```python
from build123d import *

# Parameters (mm, degrees)
SKETCH_1_R          = 2.05
SKETCH_1_R_2        = 9.525
SKETCH_1_W          = 2.1
SKETCH_1_H          = 8.1
EXTRUDE_1_DEPTH     = 2
FILLET_1_R          = 2
SKETCH_3_R          = 2.05
SKETCH_3_R_2        = 2
SKETCH_3_W          = 8.2
SKETCH_3_H          = 2.2
CUT_EXTRUDE_1_DEPTH = 2
FILLET_2_R          = 2


with BuildPart() as part:
    # 草图1 → 凸台-拉伸1 (new body)
    with BuildSketch(Plane.XY):
        with BuildLine():
            Line((230.542857143, -30.045714286), (199.556073527, -36.55591431))
            Line((199.556073527, -36.55591431), (192.746868021, -38.145714286))
            Line((192.746868021, -38.145714286), (21.365844759, -38.145714286))
            Line((21.365844759, -38.145714286), (2.692857143, -38.295714286))
            Line((2.692857143, -38.295714286), (2.692857143, -35.802553436))
            Line((2.692857143, -35.802553436), (-5.457142857, -35.802553436))
            Line((-5.457142857, -35.802553436), (-5.457142857, 41.704285714))
            Line((-5.457142857, 41.704285714), (7.542857143, 41.704285714))
            Line((7.542857143, 41.704285714), (7.542857143, 14.854285714))
            Line((7.542857143, 14.854285714), (16.542857143, 14.854285714))
            Line((16.542857143, 14.854285714), (16.542857143, 41.704285714))
            Line((16.542857143, 41.704285714), (199.542857143, 41.704285714))
            Line((199.542857143, 41.704285714), (230.542857143, 29.754285714))
            ThreePointArc((230.542857143, 29.754285714), (260.442857143, -0.145714286), (230.542857143, -30.045714286))
        make_face()
        with Locations((0.542857143, 29.854285714)):
            Circle(SKETCH_1_R, mode=Mode.SUBTRACT)
        with Locations((0.542857143, -0.145714286)):
            Circle(SKETCH_1_R, mode=Mode.SUBTRACT)
        with Locations((0.542857143, -30.145714286)):
            Circle(SKETCH_1_R, mode=Mode.SUBTRACT)
        with Locations((230.542857143, -0.145714286)):
            Circle(SKETCH_1_R_2, mode=Mode.SUBTRACT)
        with Locations((0.542857143, 14.854285714)):
            Rectangle(SKETCH_1_W, SKETCH_1_H, mode=Mode.SUBTRACT)
        with BuildLine():
            Line((59.099206329, 22.4106349), (50.542857143, 30.966984086))
            Line((50.542857143, 30.966984086), (19.430158771, -0.145714286))
            Line((19.430158771, -0.145714286), (50.542857143, -31.258412658))
            Line((50.542857143, -31.258412658), (81.655555515, -0.145714286))
            Line((81.655555515, -0.145714286), (73.099206329, 8.4106349))
            ThreePointArc((73.099206329, 8.4106349), (74.584487703, 23.895916275), (59.099206329, 22.4106349))
        make_face(mode=Mode.SUBTRACT)
        with Locations((0.542857143, -15.145714286)):
            Rectangle(SKETCH_1_W, SKETCH_1_H, mode=Mode.SUBTRACT)
    extrude(amount=EXTRUDE_1_DEPTH)

    # 圆角1
    fillet_1_edges = [part.edges().sort_by_distance(p)[0] for p in [
        (7.542857143, 41.704285714, 1),
        (7.542857143, 14.854285714, 1),
        (16.542857143, 14.854285714, 1),
        (16.542857143, 41.704285714, 1),
    ]]
    fillet(fillet_1_edges, radius=FILLET_1_R)

    # 草图3 → 切除-拉伸1 (cut)
    with BuildSketch(Plane.XY.offset(2)):
        with Locations((25.542857143, 35.704285714)):
            Circle(SKETCH_3_R)
        with Locations((110.542857143, 35.704285714)):
            Circle(SKETCH_3_R)
        with Locations((195.542857143, 35.704285714)):
            Circle(SKETCH_3_R)
        with Locations((110.542857143, -34.295714286)):
            Circle(SKETCH_3_R)
        with Locations((195.542857143, -34.295714286)):
            Circle(SKETCH_3_R)
        with Locations((25.542857143, -34.295714286)):
            Circle(SKETCH_3_R)
        with Locations((190.542857143, -0.145714286)):
            Circle(SKETCH_3_R_2)
        with Locations((140.542857143, 16.354285714)):
            Circle(SKETCH_3_R_2)
        with Locations(Location((140.542857143, -16.645714286, 0), (0, 0, 180))):
            Circle(SKETCH_3_R_2)
        with Locations((199.574018739, 19.704285714)):
            Circle(SKETCH_3_R)
        Polygon((148.153334198, 25.704285714), (148.153334198, 9.632158315), (167.669488896, 25.704285714), align=None)
        Polygon((185.542857143, -24.295714286), (138.41622539, -24.295714286), (185.542857143, 14.51445304), align=None)
        Polygon((120.542857143, -13.105881612), (120.542857143, 25.704285714), (134.014872528, 25.704285714), (134.014872528, -2.011280706), align=None)
        with Locations((184.574018739, 19.704285714)):
            Rectangle(SKETCH_3_W, SKETCH_3_H)
    extrude(amount=-CUT_EXTRUDE_1_DEPTH, mode=Mode.SUBTRACT)

    # 圆角2
    fillet_2_edges = [part.edges().sort_by_distance(p)[0] for p in [
        (167.669488896, 25.704285714, 1),
        (148.153334198, 9.632158315, 1),
        (148.153334198, 25.704285714, 1),
        (120.542857143, 25.704285714, 1),
        (134.014872528, 25.704285714, 1),
        (134.014872528, -2.011280706, 1),
        (120.542857143, -13.105881612, 1),
        (185.542857143, 14.51445304, 1),
        (185.542857143, -24.295714286, 1),
        (138.41622539, -24.295714286, 1),
    ]]
    fillet(fillet_2_edges, radius=FILLET_2_R)


solid = part.part
```
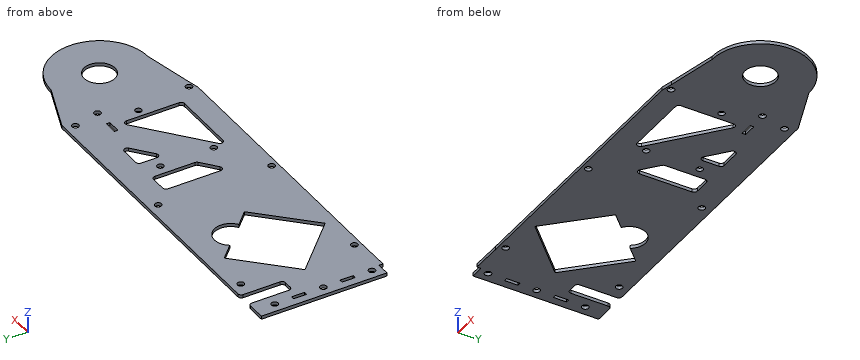
Can you work these out from the model? Positions are in its coordinate system, mm. Coordinates: 2 decimals unless noted, no trailing zeros. Write each loop counter-clockwise with the first axis right and the second up, starting at its lowest first coordinate (ties: lowest second). Pieces come first, ordered by that corner, then holes. Notation, with made-up numbers: M 5,62.25 L 10,62.25 A27 cw 10,93.25 Z; hole C -28,-32.5 d5. An arc over 180 degrees is marked long. Write item = value, one per line. Start each with the question number.
Q1. If we section it at C-C, the plane x = 218.5: Write out the boundary of the cut face in (y, z).
Q2. If we section it at B-B, the plane z = 1.6: State how many separate pieces and enclosed holes the cut face has, then the cut area to 3 significant figures.
Q3. If we section it at A-A, the plane x = 46: Write out the boundary of the cut face in (y, z), then the cut area to 3 significant figures.
Q4. I'm going to push flat-ended pins straight in: pin 1 (12 mm diameter, centred on x = 47.5, y = 27.5, fed in from -Z); pin 2 (3.5 mm diameter, centred on x = 110.54, y = 35.7, fed in from +Z); pin 3 (1 mm diameter, centred on x = 0.5, z = 1, fed in from -Y); pin 4 (0.6 mm diameter, centred on y = -37.5, z = 1.5, fed in from -X). Where does each tip first touch, or does it pass through?
Q5. If I drill on L1, parallel to X at y = 22, z = 1.7; L2, parallel to X at y = 2.5, z = 1.3; L3, parallel to X at y = -22.5, z = 0.4, over which ranges is the centre line in solid material (lowest first)? Write a range as [from, to].
Check sheet entries:
q1.outline = M -32.58,0 L 34.4,0 L 34.4,2 L -32.58,2 Z
q2.separate_pieces = 1
q2.enclosed_holes = 21
q2.area = 15,500 mm²
q3.outline = M -38.15,0 L -26.72,0 L -26.72,2 L -38.15,2 Z; M 26.42,0 L 41.7,0 L 41.7,2 L 26.42,2 Z
q3.area = 53.4 mm²
q4.pin_1 = 0
q4.pin_2 = through
q4.pin_3 = -35.8
q4.pin_4 = 2.69
q5.L1 = [-5.46, 7.54], [16.54, 41.58], [76.07, 120.54], [134.01, 148.15], [163.17, 250.63]
q5.L2 = [-5.46, 22.08], [79.01, 120.54], [134.01, 170.95], [185.54, 221.39], [239.69, 260.33]
q5.L3 = [-5.46, 41.78], [59.3, 142], [185.53, 250.4]
